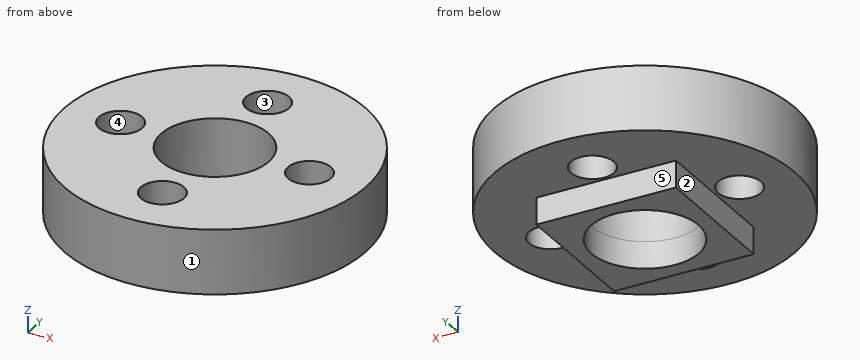
```python
from build123d import *

# Parameters (mm, degrees)
SKETCH1_R           = 17.78
SKETCH1_R_2         = 2.54
SKETCH1_R_3         = 6.35
BOSS_EXTRUDE1_DEPTH = 7.62
BOSS_EXTRUDE2_START = 3.175
SKETCH2_W           = 16.51
SKETCH2_H           = 16.51
SKETCH2_R           = 6.35
BOSS_EXTRUDE2_DEPTH = 3.175


with BuildPart() as part:
    # Sketch1 → Boss-Extrude1 (new body)
    with BuildSketch(Plane.XY):
        with Locations(Location((0, 0, 0), (0, 0, 180))):
            Circle(SKETCH1_R)
        with Locations(Location((-11.176, 0, 0), (0, 0, 180))):
            Circle(SKETCH1_R_2, mode=Mode.SUBTRACT)
        with Locations(Location((0, -11.176, 0), (0, 0, 180))):
            Circle(SKETCH1_R_2, mode=Mode.SUBTRACT)
        with Locations(Location((11.176, 0, 0), (0, 0, 180))):
            Circle(SKETCH1_R_2, mode=Mode.SUBTRACT)
        with Locations(Location((0, 11.176, 0), (0, 0, 180))):
            Circle(SKETCH1_R_2, mode=Mode.SUBTRACT)
        with Locations(Location((0, 0, 0), (0, 0, 180))):
            Circle(SKETCH1_R_3, mode=Mode.SUBTRACT)
    extrude(amount=BOSS_EXTRUDE1_DEPTH)

    # Sketch2 → Boss-Extrude2 (add)
    with BuildSketch(Plane(origin=(0, 0, 0), x_dir=(-1, 0, 0), z_dir=(0, 0, -1)).offset(BOSS_EXTRUDE2_START)):
        Rectangle(SKETCH2_W, SKETCH2_H)
        Circle(SKETCH2_R, mode=Mode.SUBTRACT)
    extrude(amount=-BOSS_EXTRUDE2_DEPTH)


solid = part.part
```
Verification items for the finished model (mm, model axes). Face numbers are marked on the shaded views. A direction names the side the tool comes from. Round coordinates to 2 decimals unless told otherwise and drop trailing zeros. Order: outer loops, then holes, each group sorted by start corner. A loop starts at its lowest first (then second) coordinate and runs counter-clockwise, first axis right, second up. Notation, with made-up numbers: (28.25, -35) -> (60.25, -35) arc R32 cw to (60.25, -5) -> close; hole circle Ø4 at (0.5, 26.25). An arc over 180 degrees is marked (long way). Put each result on its own line as item: value. Start each with the question number.
(1) Draft check along X on the marked faces 1, 2 and 3. Enter one of: +X half, -X half, draft (parallel to the pull), parting line (faces both ways), or undercut.
(2) Depth check by flat-ended pin: pin 1 Ø5 at (y, z) = (10.5, 3.5) entering from +X; pin 2 Ø8 at (x, y) = (-5, 12.5) entering from -Z; pin 3 Ø1.5 at (y, z) = (-6.5, 1) entering from +X. Enter the tip coordinate at first touch or a pass-through.
(3) Tool access check on the marked faces 4 and 5. Record the directions out of +Z, -Z, +X, -X, +Y, -Y that give a thin tool (end or side, any length) a straight path to the whole face; none if there is none.
(4) Section check A-A (x = 0). Enter the section's corners in (y, z) (3 decimals).
(5) Section check D-D (y = 13). Enter the section's corners in (x, z), then the cut area to 3 significant figures.
(6) Section check C-C (z = -1.5). Enter the section's corners in (x, y) (3 decimals).
(7) Material ranges on line 1 along Y through (x, z) = (0, 6); line 2 along X through (y, z) = (-1, 0.5); line 3 along Y through (x, z) = (2, 2), recorded low to high.
Completed:
1. face 1: parting line
1. face 2: -X half
1. face 3: undercut
2. pin 1: stops at x = 15.88
2. pin 2: stops at z = 0
2. pin 3: stops at x = 16.82
3. face 4: +Z, -Z
3. face 5: -Z, +X, -X, +Y
4. outline: (-17.78, 0) -> (-13.716, 0) -> (-13.716, 7.62) -> (-17.78, 7.62) -> close; (-8.636, 0) -> (-8.255, 0) -> (-8.255, -3.175) -> (-6.35, -3.175) -> (-6.35, 7.62) -> (-8.636, 7.62) -> close; (6.35, -3.175) -> (8.255, -3.175) -> (8.255, 0) -> (8.636, 0) -> (8.636, 7.62) -> (6.35, 7.62) -> close; (13.716, 0) -> (17.78, 0) -> (17.78, 7.62) -> (13.716, 7.62) -> close
5. outline: (-12.13, 0) -> (-1.77, 0) -> (-1.77, 7.62) -> (-12.13, 7.62) -> close; (1.77, 0) -> (12.13, 0) -> (12.13, 7.62) -> (1.77, 7.62) -> close
5. area: 158 mm2
6. outline: (-8.255, -8.255) -> (8.255, -8.255) -> (8.255, 8.255) -> (-8.255, 8.255) -> close; hole circle Ø12.7 at (0, 0)
7. line 1: y = -17.78 to -13.72, -8.64 to -6.35, 6.35 to 8.64, 13.72 to 17.78
7. line 2: x = -17.75 to -13.51, -8.84 to -6.27, 6.27 to 8.84, 13.51 to 17.75
7. line 3: y = -17.67 to -12.74, -9.61 to -6.03, 6.03 to 9.61, 12.74 to 17.67
